Here's how the part is built. I have some questions about the finished solid (model axes, mm). Give positions to 0.01 mm unless a question says otherwise; leave off trailing zeros. Write each loop counter-clockwise with the first axis right and the second up, starting at its lowest first coordinate (ties: lowest second). Pieces come first, ordered by that corner, then holes. Notation, with made-up numbers: (54, 1.25) -> (79, 1.25) arc R26 cw to (79, 19.25) -> close; hole circle Ø5 at (-4, 39.5). An arc over 180 degrees is marked (long way). Use one line per item in the form item = value.
```python
from build123d import *

# Parameters (mm, degrees)
SKETCH_1_R      = 1.5
EXTRUDE_1_DEPTH = 2.5
FILLET_1_R      = 0.2


with BuildPart() as part:
    # 草图1 → 凸台-拉伸1 (new body)
    with BuildSketch(Plane.XY):
        Polygon((1.58771324, -2.75), (3.175426481, 0), (1.58771324, 2.75), (-1.58771324, 2.75), (-3.175426481, 0), (-1.58771324, -2.75), align=None)
        Circle(SKETCH_1_R, mode=Mode.SUBTRACT)
    extrude(amount=EXTRUDE_1_DEPTH)

    # 圆角1
    fillet_1_edges = [part.edges().sort_by_distance(p)[0] for p in [
        (2.38156986, 1.375, 2.5),
        (0, 2.75, 2.5),
        (-1.5, 0, 0),
        (-2.38156986, 1.375, 2.5),
        (-2.38156986, -1.375, 2.5),
        (0, -2.75, 2.5),
        (-2.38156986, -1.375, 0),
        (-2.38156986, 1.375, 0),
        (0, 2.75, 0),
        (2.38156986, 1.375, 0),
        (2.38156986, -1.375, 0),
        (0, -2.75, 0),
        (2.38156986, -1.375, 2.5),
    ]]
    fillet(fillet_1_edges, radius=FILLET_1_R)


solid = part.part
```
Q1. Will this pin go through, and if not, where does the flat tip stop? pin 1 Ø1.5 at (y, z) = (-1, 2) entering from +X.
Result set:
pin_1 = 3.03
Q2. I want a section at B-B, the plane z = 1.15. Write out the boundary of the cut face in (x, y).
Result set:
outline = (-3.18, 0) -> (-1.59, -2.75) -> (1.59, -2.75) -> (3.18, 0) -> (1.59, 2.75) -> (-1.59, 2.75) -> close; hole circle Ø3 at (0, 0)
Q3. If we mould it in two halves opening along Y, with no side actions, what happens to faces 1 (the face through (-1.5, 0.07, 1.33)), 2 (the face through (2.32, 1.37, 2.44)), 3 (the face through (0, 2, 0))? For each: +Y half, -Y half, draft (parallel to the pull), parting line (faces both ways), or undercut.
Result set:
face_1 = undercut
face_2 = +Y half
face_3 = draft
Q4. I want a section at A-A, the plane x = 0. Write out the boundary of the cut face in (y, z).
Result set:
outline = (-2.75, 0.2) arc R0.2 ccw to (-2.55, 0) -> (-1.7, 0) arc R0.2 ccw to (-1.5, 0.2) -> (-1.5, 2.5) -> (-2.55, 2.5) arc R0.2 ccw to (-2.75, 2.3) -> close; (1.5, 0.2) arc R0.2 ccw to (1.7, 0) -> (2.55, 0) arc R0.2 ccw to (2.75, 0.2) -> (2.75, 2.3) arc R0.2 ccw to (2.55, 2.5) -> (1.5, 2.5) -> close
Q5. If I drill on line 1 along Y through (x, z) = (0, 0.9); line 2 along Y through (x, z) = (-0.5, 0.9); line 3 along X through (y, z) = (1.05, 1.7), over which ranges is the centre line in solid material (lowest first)? Write a range as from..to.
Result set:
line_1 = -2.75..-1.5, 1.5..2.75
line_2 = -2.75..-1.41, 1.41..2.75
line_3 = -2.57..-1.07, 1.07..2.57
